```python
from build123d import *


with BuildPart() as f1:
    # F0 (on Right) → F1 (revolve)
    with BuildSketch(Plane.YZ):
        with BuildLine():
            Line((0, 25), (0, 0))
            Line((0, 0), (88, 0))
            Line((88, 0), (88, 16))
            Line((88, 16), (85, 16))
            Line((85, 16), (85, 20))
            Line((85, 20), (68, 20))
            Line((68, 20), (68, 31))
            Line((68, 31), (56, 31))
            ThreePointArc((56, 31), (50, 25), (44, 31))
            Line((44, 31), (6, 31))
            ThreePointArc((6, 31), (1.757359, 29.242641), (0, 25))
        make_face()
    revolve(axis=Axis((0, 61.81017, 0), (0, 1, 0)))

    # F2 (on Right) → F3 (revolve, cut)
    with BuildSketch(Plane.YZ):
        Polygon((13.5, 12.5), (13.5, 16), (1.5, 16), (1.5, 0), (88, 0), (88, 6), (30, 6), (30, 16), (22, 16), (22, 20.5), (16.5, 20.5), (16.5, 12.5), align=None)
        Polygon((1.5, 0), (1.5, 16), (1.5, 25), (0, 25), (0, 0), align=None)
    revolve(axis=Axis((0, 44, 0), (0, -1, 0)), mode=Mode.SUBTRACT)


solid = f1.part
```
Verification items for the finished model (mm, model axes). A direction names the side the tool comes from. Give positions to 0.01 mm unless a question says otherwise; leave off trailing zeros. Order: outer loops, then holes, each group sorted by start corner. A loop starts at its lowest first (then second) coordinate and runs counter-clockwise, first axis right, second up. Notation, with made-up numbers: (56.5, 13) -> (74.5, 13) arc R23 cw to (74.5, 30) -> close; hole circle Ø3 at (83, -24.75). An arc over 180 degrees is marked (long way). One line per item, written item: value.
(1) Sectioned sample at B-B on y = 65.5. Record the cut outline in (x, z), then the cut area to 3 significant figures.
Final values:
outline: circle Ø62 at (0, 0); hole circle Ø12 at (0, 0)
area: 2,910 mm^2
(2) Draft check along Z on faces 5 (the face through (30.736, 61.916, -4.036)), 6 (the face through (13.43, 85, 8.98)), 7 (the face through (11, 22, -12)). Enter one of: pulls with the +Z half, pulls with the -Z half, needs draft (parallel to the pull), parting line crosses it, or undercut.
Final values:
face 5: parting line crosses it
face 6: needs draft
face 7: undercut
(3) Sectioned sample at A-A on y = 79. Record the cut outline in (x, z), then the cut area to 3 significant figures.
Final values:
outline: circle Ø40 at (0, 0); hole circle Ø12 at (0, 0)
area: 1,140 mm^2
(4) Gauge pin test, flat ends, axial feed: pin 1 (12 mm diameter, centred on x = -19, z = -23.5, fed in from +Y); pin 2 (1.5 mm diameter, centred on y = 26.5, z = -4.5, fed in from +X); pin 3 (1 mm diameter, centred on x = -9, z = -22, fed in from -Y). Record the tip position at first contact, or that the pin passes through.
Final values:
pin 1: y = 68
pin 2: x = 30.77
pin 3: y = 1.5
(5) Scan lines: line 1 along X through (y, z) = (9.5, 0); line 2 along Y through (x, z) = (-4.5, 15); line 3 along Y through (x, z) = (-7.5, 15). Record each from-to range of solid material in increasing order. Write a range as [from, to].
Final values:
line 1: [-31, -16], [16, 31]
line 2: [13.5, 16.5], [30, 88]
line 3: [1.5, 16.5], [22, 85]
(6) Tool access check on faces 1 (the face through (-20.2, 68, 0.4)), 2 (the face through (-7.509, 0.74, 23.846)), 3 (the face through (9, 16.5, -9)), 4 (the face through (30.736, 24.734, -4.036)). Record the directions out of +Z, -Z, +X, -X, +Y, -Y that give a thin tool (end or side, any length) a straight path to the whole face; none if there is none.
Final values:
face 1: +Y
face 2: -Y
face 3: none
face 4: +Y, -Y
